For this review, take the finished solid that the model builds, in its own axes (mm). Give positions to 0.01 mm unless a question says otherwise; leave off trailing zeros. Write each loop counter-clockwise with the first axis right and the second up, starting at its lowest first coordinate (ties: lowest second). Pieces come first, ordered by that corner, then holes. Notation, with made-up numbers: M -28,66 L 21,66 A20 cw 21,78 Z; hole C 38.25,63.25 d8. An arc over 180 degrees is marked long. Write item = value, one per line.
```python
from build123d import *

# Parameters (mm, degrees)
BOSS_EXTRUDE1_START = 56.6115
SKETCH2_R           = 1.5635
SKETCH2_R_2         = 5
BOSS_EXTRUDE1_DEPTH = 6


with BuildPart() as part:
    # Sketch2 → Boss-Extrude1 (new body)
    with BuildSketch(Plane.XY.offset(BOSS_EXTRUDE1_START)):
        with BuildLine():
            Line((300, 27.5), (-84.125211865, 27.5))
            ThreePointArc((-84.125211865, 27.5), (-167, 0), (-84.125211865, -27.5))
            Line((-84.125211865, -27.5), (300, -27.5))
            ThreePointArc((300, -27.5), (327.5, 0), (300, 27.5))
        make_face()
        with Locations((0, 22.5)):
            Circle(SKETCH2_R, mode=Mode.SUBTRACT)
        with Locations((22.5, 0)):
            Circle(SKETCH2_R, mode=Mode.SUBTRACT)
        with Locations((0, -22.5)):
            Circle(SKETCH2_R, mode=Mode.SUBTRACT)
        with Locations((-22.5, 0)):
            Circle(SKETCH2_R, mode=Mode.SUBTRACT)
        with Locations((-121, -22.5)):
            Circle(SKETCH2_R, mode=Mode.SUBTRACT)
        with Locations((-143.5, 0)):
            Circle(SKETCH2_R, mode=Mode.SUBTRACT)
        with Locations((-121, 22.5)):
            Circle(SKETCH2_R, mode=Mode.SUBTRACT)
        with Locations((-98.5, 0)):
            Circle(SKETCH2_R, mode=Mode.SUBTRACT)
        Circle(SKETCH2_R_2, mode=Mode.SUBTRACT)
    extrude(amount=BOSS_EXTRUDE1_DEPTH)


solid = part.part
```
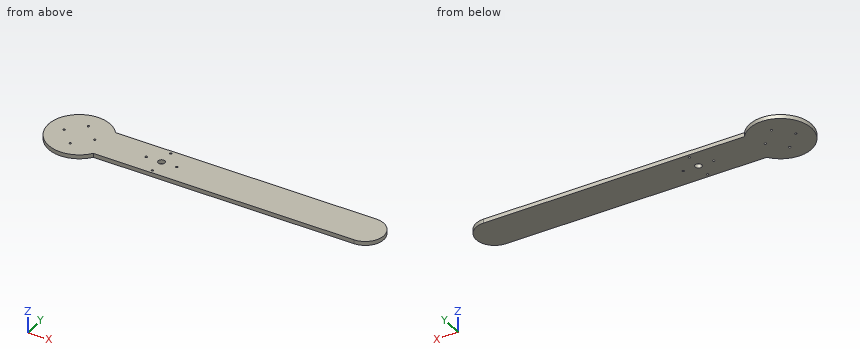
1. We need section A-A, the plane z = 58.75. Count the separate pieces of the cut face and the enclosed holes in it, then the cut area to 3 significant figures.
Responses:
separate_pieces = 1
enclosed_holes = 9
area = 28,500 mm2
2. We need section B-B, the plane x = 273. Write out the cut boundary in (y, z).
Responses:
outline = M -27.5,56.61 L 27.5,56.61 L 27.5,62.61 L -27.5,62.61 Z
3. Insertion check: P1, Ø1.5, axis at y = -18, z = 60.5, coming from the -X side. The pin has a flat end and moves straight along its axis. Give the tip position at first contact, or say it passes through.
Responses:
P1 = -163.64
4. For line 1 along Y through (x, z) = (0, 58.5); line 2 along Y through (x, z) = (-22.5, 58.8); line 3 along Y through (x, z) = (154.5, 60.65), list the stretches that pass through material, from the lowest coordinate up. Write a range as from..to.
Responses:
line_1 = -27.5..-24.06, -20.94..-5, 5..20.94, 24.06..27.5
line_2 = -27.5..-1.56, 1.56..27.5
line_3 = -27.5..27.5
